Geometry: see drawing. Coordinates: mm, zero at the bounding-box minimum. A direction names the side the tool comes from. Give positions to 0.01 mm unless a question says otherwise; leave off trailing zeros. Loops run counter-clockwise (first coordinate to the right, second up) from the corner with the lowest first, then second, coordinate; pieces in that order, holes last. Notation, with made-up numbers: M 55.5,32.25 L 93.5,32.25 A27 cw 93.5,61.25 Z; hole C 87,14.25 d2. An arc over 180 degrees is marked long. Put each result on its own line as item: value.
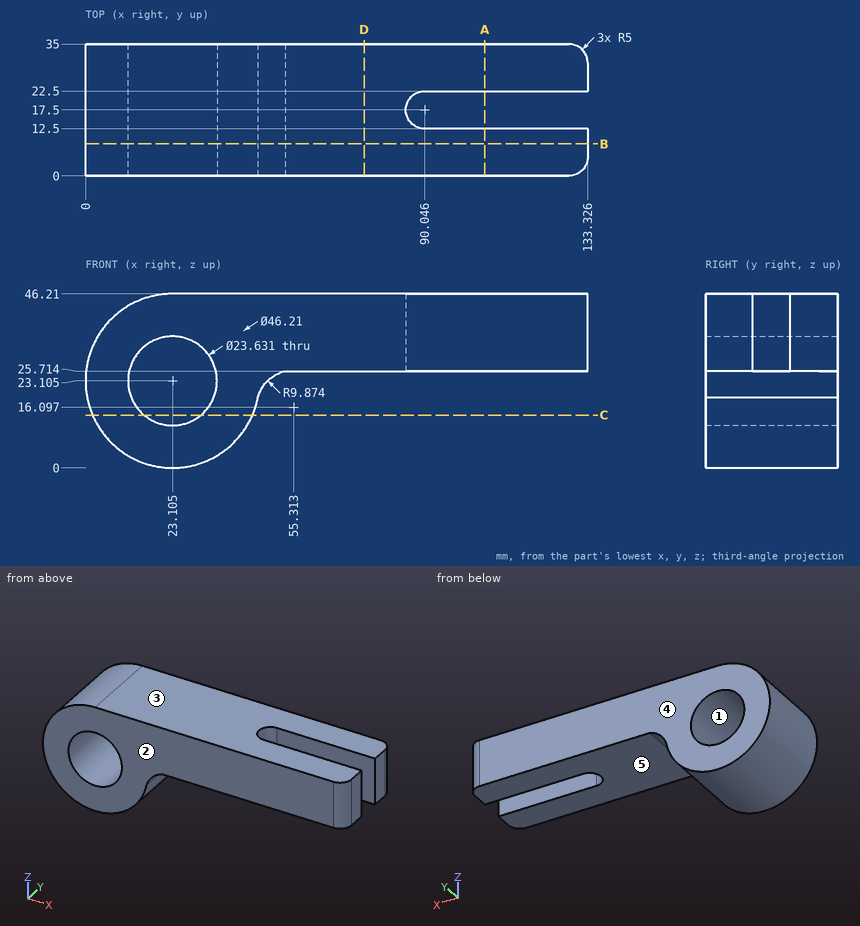
1. Section query B-B (y = 8.5). Output: boundary loops of the cut face in (x, z) (1 decimal), plus the area to 3 significant figures.
Found:
outline: M 23.1,46.2 A23.1 ccw long 45.8,18.7 A9.9 cw 53.1,25.7 L 133.3,25.7 L 133.3,46.2 Z; hole C 23.1,23.1 d23.6
area: 3,150 mm^2
2. Draft query along Z for the marked faces 1, 2 and 3. Return one class per face: pulls with the +Z half, pulls with the -Z half, needs draft (parallel to the pull), parting line crosses it, or undercut.
Found:
face 1: undercut
face 2: needs draft
face 3: pulls with the +Z half
3. Contact query for flat-ended pins moving along their axis: P1, Ø5, axis at x = 16.5, y = 19.5, coming from the -Z side; P2, Ø10.5, axis at x = 105.5, y = 24.5, coming from the -Z side; P3, Ø5, axis at y = 12, z = 21.5, coming from the -X side. Output: stop coordinate, or through.
Found:
P1: z = 0.37
P2: z = 25.71
P3: x = 0
4. Section query C-C (z = 14). Output: boundary loops of the cut face in (x, y) (1 decimal).
Found:
outline: M 1.9,0 L 15.6,0 L 15.6,35 L 1.9,35 Z; M 30.6,0 L 44.3,0 L 44.3,35 L 30.6,35 Z
5. Section query D-D (x = 74). Output: boundary loops of the cut face in (y, z) (1 decimal), plus the area to 3 significant figures.
Found:
outline: M 0,25.7 L 35,25.7 L 35,46.2 L 0,46.2 Z
area: 717 mm^2
6. Access query for the marked faces 4 and 5. Directions: +Z, -Z, +X, -X, +Y, -Y. A direction counts if a zero-diameter tool reaches every point of the face in a straight line with its end or side. Return the directions, or none.
Found:
face 4: +Z, -Z, +X, -X, +Y
face 5: -Z, +X, +Y, -Y
7. Material intervals for line 1 (Y direction, x = 104.5, z = 26); line 2 (Z direction, x = 57, y = 6) (1 decimal); line 3 (Z direction, x = 16.5, y = 6) (1 decimal), sorted ascending. Write a range as from..to.
Found:
line 1: 0..12.5, 22.5..35
line 2: 25.7..46.2
line 3: 1..13.3, 32.9..45.2
8. Section query A-A (x = 106). Output: boundary loops of the cut face in (y, z) (1 decimal).
Found:
outline: M 0,25.7 L 12.5,25.7 L 12.5,46.2 L 0,46.2 Z; M 22.5,25.7 L 35,25.7 L 35,46.2 L 22.5,46.2 Z
